from build123d import *

# Parameters (mm, degrees)
SKETCH_1_W           = 30
SKETCH_1_H           = 12
SKETCH_1_R           = 1.56
EXTRUDE_1_DEPTH      = 3
SKETCH_2_W           = 13
SKETCH_2_H           = 12
EXTRUDE_2_DEPTH      = 3
EXTRUDE_3_DEPTH      = 2
EXTRUDE_3_DEPTH_BACK = 2
SKETCH_8_W           = 8
SKETCH_8_H           = 8
SKETCH_8_R           = 2
EXTRUDE_4_DEPTH      = 2
CHAMFER_3_SIZE       = 1.945839098
CHAMFER_3_SIZE_2     = 1
CHAMFER_6_SIZE       = 1


with BuildPart() as part:
    # 草图1 → 凸台-拉伸1 (new body)
    with BuildSketch(Plane.XY):
        with Locations((15, 6)):
            Rectangle(SKETCH_1_W, SKETCH_1_H)
        with Locations((5.625, 6)):
            Circle(SKETCH_1_R, mode=Mode.SUBTRACT)
        with Locations((24.375, 6)):
            Circle(SKETCH_1_R, mode=Mode.SUBTRACT)
    extrude(amount=EXTRUDE_1_DEPTH)

    # 草图2 → 凸台-拉伸2 (add)
    with BuildSketch(Plane.XY.offset(3)):
        with Locations((15, 6)):
            Rectangle(SKETCH_2_W, SKETCH_2_H)
    extrude(amount=EXTRUDE_2_DEPTH)

    # 草图4 → 凸台-拉伸3 (add, two sides: drawn at the far end of the back side and taken through both)
    with BuildSketch(Plane(origin=(15, 0, 0), x_dir=(0, 0, -1), z_dir=(1, 0, 0)).offset(-EXTRUDE_3_DEPTH_BACK)):
        Polygon((-3, 0), (-24.650635095, -9.5), (-24.650635095, -6.5), (-3, 12), (-3, 6), align=None)
    extrude(amount=EXTRUDE_3_DEPTH + EXTRUDE_3_DEPTH_BACK)

    # 草图8 → 凸台-拉伸4 (add)
    with BuildSketch(Plane.XY.offset(24.650635095)):
        with Locations((15, -10.5)):
            Rectangle(SKETCH_8_W, SKETCH_8_H)
        with Locations((15, -11.7)):
            Circle(SKETCH_8_R, mode=Mode.SUBTRACT)
    extrude(amount=EXTRUDE_4_DEPTH)

    # 倒角3
    # the kernel refuses this chamfer: 1.945839098, 1 mm, written as the material it adds along each edge
    with BuildSketch(Plane(origin=(17, -9.5, 24.650635095), x_dir=(0, -0.9999018246669207, 0.014012174269630025), z_dir=(-1, 0, 0))) as chamfer_3_piece_1_section:
        Polygon((CHAMFER_3_SIZE * 0.999901824771, -CHAMFER_3_SIZE * 0.0140121742711), (-CHAMFER_3_SIZE_2 * 0.414599028562, -CHAMFER_3_SIZE_2 * 0.910004200823), (0, 0), align=None)
    chamfer_3_piece_1 = extrude(amount=4, mode=Mode.PRIVATE)
    chamfer_3_piece_1 = chamfer_3_piece_1 - Plane(origin=(15, -11.7, 24.270363883), x_dir=(1, 0, 0), z_dir=(0, 0, -1)) * Cylinder(2, 16, mode=Mode.PRIVATE)
    add(chamfer_3_piece_1)
    # the kernel refuses this chamfer: 1.945839098, 1 mm, written as the material it adds along each edge
    with BuildSketch(Plane(origin=(17, -14.017522086, 24.650635095), x_dir=(-0.027495876610585647, 0, -0.9996219169112968), z_dir=(0, 1, 0))) as chamfer_3_2_piece_1_section:
        Polygon((CHAMFER_3_SIZE_2 * 0.999621916911, -CHAMFER_3_SIZE_2 * 0.0274958766106), (-CHAMFER_3_SIZE_2 * 0.0274958766106, -CHAMFER_3_SIZE_2 * 0.999621916911), (0, 0), align=None)
    chamfer_3_2_piece_1 = extrude(amount=7.517522086, mode=Mode.PRIVATE)
    chamfer_3_2_piece_1 = split(chamfer_3_2_piece_1, bisect_by=Plane(origin=(17.387306177, -10.236604408, 24.178960298), z_dir=(0, 0.3633942713145685, 0.9316354456415631)), keep=Keep.TOP, mode=Mode.PRIVATE)
    chamfer_3_2_piece_1 = split(chamfer_3_2_piece_1, bisect_by=Plane(origin=(17.387306177, -9.521448323, 24.699516127), z_dir=(0, -0.9157242946977782, -0.4018071877160198)), keep=Keep.TOP, mode=Mode.PRIVATE)
    add(chamfer_3_2_piece_1)
    with BuildSketch(Plane(origin=(17, -14.017522086, 24.650635095), x_dir=(-0.027495876610585647, 0, -0.9996219169112968), z_dir=(0, 1, 0))) as chamfer_3_2_piece_2_section:
        Polygon((CHAMFER_3_SIZE_2 * 0.999621916911, -CHAMFER_3_SIZE_2 * 0.0274958766106), (-CHAMFER_3_SIZE_2 * 0.0274958766106, -CHAMFER_3_SIZE_2 * 0.999621916911), (0, 0), align=None)
    chamfer_3_2_piece_2 = extrude(amount=7.517522086, mode=Mode.PRIVATE)
    chamfer_3_2_piece_2 = split(chamfer_3_2_piece_2, bisect_by=Plane(origin=(16.988383788, -8.994550798, 23.694484135), z_dir=(0, -0.3633942713145685, -0.9316354456415631)), keep=Keep.TOP, mode=Mode.PRIVATE)
    chamfer_3_2_piece_2 = split(chamfer_3_2_piece_2, bisect_by=Plane(origin=(16.988383788, -9.059659256, 23.647092278), z_dir=(0, 0.9157242946977782, 0.4018071877160198)), keep=Keep.TOP, mode=Mode.PRIVATE)
    add(chamfer_3_2_piece_2)
    with BuildSketch(Plane(origin=(17, -14.017522086, 24.650635095), x_dir=(-0.027495876610585647, 0, -0.9996219169112968), z_dir=(0, 1, 0))) as chamfer_3_2_piece_3_section:
        Polygon((CHAMFER_3_SIZE_2 * 0.999621916911, -CHAMFER_3_SIZE_2 * 0.0274958766106), (-CHAMFER_3_SIZE_2 * 0.0274958766106, -CHAMFER_3_SIZE_2 * 0.999621916911), (0, 0), align=None)
    chamfer_3_2_piece_3 = extrude(amount=7.517522086, mode=Mode.PRIVATE)
    chamfer_3_2_piece_3 = split(chamfer_3_2_piece_3, bisect_by=Plane(origin=(17.33510096, -8.285636608, 23.417964648), z_dir=(0, 0.3633942713145685, 0.9316354456415631)), keep=Keep.TOP, mode=Mode.PRIVATE)
    chamfer_3_2_piece_3 = split(chamfer_3_2_piece_3, bisect_by=Plane(origin=(17.33510096, -9.12878782, 23.804637257), z_dir=(0, 0.9157242946977782, 0.4018071877160198)), keep=Keep.TOP, mode=Mode.PRIVATE)
    chamfer_3_2_piece_3 = split(chamfer_3_2_piece_3, bisect_by=Plane(origin=(17.33510096, -6.945348717, 25.171828747), z_dir=(0, -0.7602566248543531, -0.649622863179143)), keep=Keep.TOP, mode=Mode.PRIVATE)
    add(chamfer_3_2_piece_3)
    with BuildSketch(Plane(origin=(17, -14.017522086, 24.650635095), x_dir=(-0.027495876610585647, 0, -0.9996219169112968), z_dir=(0, 1, 0))) as chamfer_3_2_piece_4_section:
        Polygon((CHAMFER_3_SIZE_2 * 0.999621916911, -CHAMFER_3_SIZE_2 * 0.0274958766106), (-CHAMFER_3_SIZE_2 * 0.0274958766106, -CHAMFER_3_SIZE_2 * 0.999621916911), (0, 0), align=None)
    chamfer_3_2_piece_4 = extrude(amount=10.089205074, mode=Mode.PRIVATE)
    chamfer_3_2_piece_4 = split(chamfer_3_2_piece_4, bisect_by=Plane(origin=(17.227791028, -6.5, 24.129350329), z_dir=(0, 1, 0)), keep=Keep.TOP, mode=Mode.PRIVATE)
    chamfer_3_2_piece_4 = split(chamfer_3_2_piece_4, bisect_by=Plane(origin=(17.227791028, -6.148560632, 24.239343986), z_dir=(0, -0.7602566248543531, -0.649622863179143)), keep=Keep.TOP, mode=Mode.PRIVATE)
    add(chamfer_3_2_piece_4)
    with BuildSketch(Plane(origin=(13, -3.928317012, 24.650635095), x_dir=(0.027495876610585647, 0, -0.9996219169112968), z_dir=(0, -1, 0))) as chamfer_3_2_piece_5_section:
        Polygon((CHAMFER_3_SIZE_2 * 0.999621916911, -CHAMFER_3_SIZE_2 * 0.0274958766106), (-CHAMFER_3_SIZE_2 * 0.0274958766106, -CHAMFER_3_SIZE_2 * 0.999621916911), (0, 0), align=None)
    chamfer_3_2_piece_5 = extrude(amount=10.089205074, mode=Mode.PRIVATE)
    chamfer_3_2_piece_5 = split(chamfer_3_2_piece_5, bisect_by=Plane(origin=(12.772208972, -6.5, 24.129350329), z_dir=(0, 1, 0)), keep=Keep.TOP, mode=Mode.PRIVATE)
    chamfer_3_2_piece_5 = split(chamfer_3_2_piece_5, bisect_by=Plane(origin=(12.772208972, -6.148560632, 24.239343986), z_dir=(0, -0.7602566248543531, -0.649622863179143)), keep=Keep.TOP, mode=Mode.PRIVATE)
    add(chamfer_3_2_piece_5)
    with BuildSketch(Plane(origin=(13, -6.5, 24.650635095), x_dir=(0.027495876610585647, 0, -0.9996219169112968), z_dir=(0, -1, 0))) as chamfer_3_2_piece_6_section:
        Polygon((CHAMFER_3_SIZE_2 * 0.999621916911, -CHAMFER_3_SIZE_2 * 0.0274958766106), (-CHAMFER_3_SIZE_2 * 0.0274958766106, -CHAMFER_3_SIZE_2 * 0.999621916911), (0, 0), align=None)
    chamfer_3_2_piece_6 = extrude(amount=7.517522086, mode=Mode.PRIVATE)
    chamfer_3_2_piece_6 = split(chamfer_3_2_piece_6, bisect_by=Plane(origin=(12.66489904, -8.285636608, 23.417964648), z_dir=(0, 0.3633942713145685, 0.9316354456415631)), keep=Keep.TOP, mode=Mode.PRIVATE)
    chamfer_3_2_piece_6 = split(chamfer_3_2_piece_6, bisect_by=Plane(origin=(12.66489904, -9.12878782, 23.804637257), z_dir=(0, 0.9157242946977782, 0.4018071877160198)), keep=Keep.TOP, mode=Mode.PRIVATE)
    chamfer_3_2_piece_6 = split(chamfer_3_2_piece_6, bisect_by=Plane(origin=(12.66489904, -6.945348717, 25.171828747), z_dir=(0, -0.7602566248543531, -0.649622863179143)), keep=Keep.TOP, mode=Mode.PRIVATE)
    add(chamfer_3_2_piece_6)
    with BuildSketch(Plane(origin=(13, -6.5, 24.650635095), x_dir=(0.027495876610585647, 0, -0.9996219169112968), z_dir=(0, -1, 0))) as chamfer_3_2_piece_7_section:
        Polygon((CHAMFER_3_SIZE_2 * 0.999621916911, -CHAMFER_3_SIZE_2 * 0.0274958766106), (-CHAMFER_3_SIZE_2 * 0.0274958766106, -CHAMFER_3_SIZE_2 * 0.999621916911), (0, 0), align=None)
    chamfer_3_2_piece_7 = extrude(amount=7.517522086, mode=Mode.PRIVATE)
    chamfer_3_2_piece_7 = split(chamfer_3_2_piece_7, bisect_by=Plane(origin=(12.612693823, -10.236604408, 24.178960298), z_dir=(0, 0.3633942713145685, 0.9316354456415631)), keep=Keep.TOP, mode=Mode.PRIVATE)
    chamfer_3_2_piece_7 = split(chamfer_3_2_piece_7, bisect_by=Plane(origin=(12.612693823, -9.521448323, 24.699516127), z_dir=(0, -0.9157242946977782, -0.4018071877160198)), keep=Keep.TOP, mode=Mode.PRIVATE)
    add(chamfer_3_2_piece_7)
    with BuildSketch(Plane(origin=(13, -6.5, 24.650635095), x_dir=(0.027495876610585647, 0, -0.9996219169112968), z_dir=(0, -1, 0))) as chamfer_3_2_piece_8_section:
        Polygon((CHAMFER_3_SIZE_2 * 0.999621916911, -CHAMFER_3_SIZE_2 * 0.0274958766106), (-CHAMFER_3_SIZE_2 * 0.0274958766106, -CHAMFER_3_SIZE_2 * 0.999621916911), (0, 0), align=None)
    chamfer_3_2_piece_8 = extrude(amount=7.517522086, mode=Mode.PRIVATE)
    chamfer_3_2_piece_8 = split(chamfer_3_2_piece_8, bisect_by=Plane(origin=(13.011616212, -8.994550798, 23.694484135), z_dir=(0, -0.3633942713145685, -0.9316354456415631)), keep=Keep.TOP, mode=Mode.PRIVATE)
    chamfer_3_2_piece_8 = split(chamfer_3_2_piece_8, bisect_by=Plane(origin=(13.011616212, -9.059659256, 23.647092278), z_dir=(0, 0.9157242946977782, 0.4018071877160198)), keep=Keep.TOP, mode=Mode.PRIVATE)
    add(chamfer_3_2_piece_8)

    # 倒角6
    chamfer_6_edges = [part.edges().sort_by_distance(p)[0] for p in [
        (15, -6.5, 26.650635095),
    ]]
    chamfer(chamfer_6_edges, length=CHAMFER_6_SIZE)


solid = part.part
Geometry: final body of the model. Coordinates: model frame, mm. A direction names the side the tool comes from. Round coordinates to 2 decimals unless told otherwise and drop trailing zeros. Order: outer loops, then holes, each group sorted by start corner. A loop starts at its lowest first (then second) coordinate and runs counter-clockwise, first axis right, second up. Notation, with made-up numbers: (40.25, -5.75) -> (59.25, -5.75) arc R20 cw to (59.25, 7.25) -> close; hole circle Ø7 at (28.5, 66). An arc over 180 degrees is marked (long way). Put each result on its own line as item: value. Start each with the question number.
Q1. First-contact query: pin 1 (5.5 mm diameter, centred on y = 2, z = 12, fed in from -X); pin 2 (5 mm diameter, centred on y = 8.5, z = 10.5, fed in from +X); pin 3 (5 mm diameter, centred on x = 15.5, z = 3.5, fed in from -Y). Flat tips, straight axial feed; report the tip coordinate or a pass-through.
Q2. Reachability of faces 5 (the cylindrical face through (6.345, 4.616, 1.479)), 6 (the flat face through (30, 6, 1)), 7 (the flat face through (15, -6.5, 25)), 8 (the flat face through (3, 6, 3)), 9 (the flat face through (27, 6, 3)) from +Z, -Z, +X, -X, +Y, -Y: full face, straight path, thin tool, end or side. Return the list, or none.
Q3. Section C-C on z = 18. Return the cut outline in (x, y).
Q4. Pull-direction query (Y, two-part tool) for faces 1 (the flat face through (14.94, -7.01, 26.16)), 2 (the flat face through (15, 0, 2)), 3 (the cylindrical face through (22.817, 6.069, 1.479)), 4 (the cylindrical face through (14.566, -9.748, 25.589)); classes: +Y half, -Y half, draft (parallel to the pull), parting line (faces both ways), or undercut.
Q5. Section A-A on x = 15. Return the cut outline in (y, z), and give its area (3 significant figures).
Q6. Section B-B on y = 6. Return the cut outline in (x, z) (3 decimals), and give its area (3 significant figures).
Q7. Line query: probe 1 along X at (y, z) = (-11.7, 26); probe 2 along X at (y, z) = (4.75, 2.5); probe 3 along Y at (x, z) = (15, 25.55). Output: solid intervals per line, ascending.
Q8. Section D-D on x = 6.75. Return the cut outline in (y, z), and give its area (3 significant figures).
Ans:
1. pin 1: stops at x = 13
1. pin 2: stops at x = 17
1. pin 3: stops at y = -1.32
2. face 5: +Z, -Z
2. face 6: +Z, -Z, +X, +Y, -Y
2. face 7: +Z, +X, -X, +Y
2. face 8: +Z, -X, +Y, -Y
2. face 9: +Z, +X, +Y, -Y
3. outline: (13, -6.58) -> (17, -6.58) -> (17, -0.82) -> (13, -0.82) -> close
4. face 1: +Y half
4. face 2: -Y half
4. face 3: undercut
4. face 4: undercut
5. outline: (-14.5, 24.65) -> (-13.7, 24.65) -> (-13.7, 26.65) -> (-14.5, 26.65) -> close; (-9.7, 23.97) -> (-9.1, 23.73) -> (0, 3) -> (0, 0) -> (12, 0) -> (12, 6) -> (9.44, 6) -> (-6.5, 24.65) -> (-6.5, 25.65) -> (-7.5, 26.65) -> (-9.7, 26.65) -> close
5. area: 210 mm2
6. outline: (0, 0) -> (4.065, 0) -> (4.065, 3) -> (0, 3) -> close; (7.185, 0) -> (22.815, 0) -> (22.815, 3) -> (21.5, 3) -> (21.5, 6) -> (17, 6) -> (17, 10.022) -> (13, 10.022) -> (13, 6) -> (8.5, 6) -> (8.5, 3) -> (7.185, 3) -> close; (25.935, 0) -> (30, 0) -> (30, 3) -> (25.935, 3) -> close
6. area: 126 mm2
7. probe 1: x = 11 to 13, 17 to 19
7. probe 2: x = 0 to 4.69, 6.56 to 23.44, 25.31 to 30
7. probe 3: y = -14.5 to -13.7, -9.7 to -6.5
8. outline: (0, 0) -> (4.92, 0) -> (4.92, 3) -> (0, 3) -> close; (7.08, 0) -> (12, 0) -> (12, 3) -> (7.08, 3) -> close
8. area: 29.5 mm2
